from build123d import *

# Parameters (mm, degrees)
F1_DEPTH = 24.314562
F2_R     = 17.41648
F3_DEPTH = 102.574684


with BuildPart() as f1:
    # F0 (on Top) → F1 (new body)
    with BuildSketch(Plane.XY):
        Polygon((-16.025186, 26.466794), (-32.313049, 0), (-18.656433, -30.649543), (25.181532, -30.649543), (33.363849, 0), (16.999215, 26.466794), align=None)
    extrude(amount=F1_DEPTH)

    # F2 (on Top) → F3 (join)
    with BuildSketch(Plane.XY):
        Circle(F2_R)
    extrude(amount=F3_DEPTH)


solid = f1.part
Verification items for the finished model (mm, model axes). A direction names the side the tool comes from. Give positions to 0.01 mm unless a question says otherwise; leave off trailing zeros. Write each loop counter-clockwise with the first axis right and the second up, starting at its lowest first coordinate (ties: lowest second). Pieces come first, ordered by that corner, then holes. Notation, with made-up numbers: (19, -29) - (50, -29) arc R14 ccw to (50, -4) - close; hole circle Ø5 at (40, -34). An arc over 180 degrees is marked (long way). Answer as CSV lines item,"result". Start each with the question number.
1. Sectioned sample at B-B (y = -8). Record the boundary of the cut face in (x, z), then the cut area to 3 significant figures.
2. Set-up check for faces 1 (the face through (-25.58, -15.11, 11.99)), 2 (the face through (-12.84, 11.77, 62.9)): record each of +Z, -Z, +X, -X, +Y, -Y from which the full face is reachable in a straight line by a thin tool's end or side.
3. Sectioned sample at A-A (x = 0). Record the boundary of the cut face in (y, z).
4. Depth check by flat-ended pin: pin 1 (3 mm diameter, centred on x = -15, z = 85.5, fed in from -Y); pin 2 (5 mm diameter, centred on y = 10.5, z = 76.5, fed in from +X); pin 3 (4 mm diameter, centred on x = -2, z = 60, fed in from +Y). Enter the tip coordinate at first touch or a pass-through.
5. Thickness scan on line 1 (Z direction, x = 12, y = 16); line 2 (Y direction, x = -28, z = 17.5); line 3 (X direction, y = -11, z = 13.5). Record the ranges inside material, lowest first.
6. Sectioned sample at C-C (z = 14). Record the boundary of the cut face in (x, y).
7. Sectioned sample at D-D (z = 83.5). Record the boundary of the cut face in (x, y), then the cut area to 3 significant figures.
Derived:
1,outline,"(-28.75, 0) - (31.23, 0) - (31.23, 24.31) - (15.47, 24.31) - (15.47, 102.57) - (-15.47, 102.57) - (-15.47, 24.31) - (-28.75, 24.31) - close"
1,area,"3,880 mm²"
2,face 1,"+Z, -Z, -X, -Y"
2,face 2,"+Z"
3,outline,"(-30.65, 0) - (26.47, 0) - (26.47, 24.31) - (17.42, 24.31) - (17.42, 102.57) - (-17.42, 102.57) - (-17.42, 24.31) - (-30.65, 24.31) - close"
4,pin 1,"y = -11"
4,pin 2,"x = 15.47"
4,pin 3,"y = 17.42"
5,line 1,"0 to 24.31"
5,line 2,"-9.68 to 7.01"
5,line 3,"-27.41 to 30.43"
6,outline,"(-32.31, 0) - (-18.66, -30.65) - (25.18, -30.65) - (33.36, 0) - (17, 26.47) - (-16.03, 26.47) - close"
7,outline,"circle Ø34.83 at (0, 0)"
7,area,"953 mm²"
